Geometry: see drawing. Coordinates: mm, zero at the bounding-box minimum. A direction names the side the tool comes from. Give positions to 0.01 mm unless a question says otherwise; leave off trailing zeros. Write each loop counter-clockwise with the first axis right and the second up, starting at its lowest first coordinate (ties: lowest second). Pieces come first, ordered by that corner, then holes. Notation, with made-up numbers: (29, 16) -> (82, 16) arc R12 ccw to (82, 38) -> close; hole circle Ø10 at (-8, 52.25). An arc over 180 degrees is marked (long way). Use one line per item in the form item = value. Start each with the question number.
(1) Cut plane D-D, the plane z = 21.25. Output: boundary loops of the cut face in (x, y).
(2) Draft query along Z for the marked faces 4, 5 and 6. Return one class per face: pulls with the +Z half, pulls with the -Z half, needs draft (parallel to the pull), parting line crosses it, or undercut.
(3) Cut plane A-A, the plane z = 10.75. Output: boundary loops of the cut face in (x, y) (1 decimal).
(4) Cut plane C-C, the plane x = 18.75. Output: boundary loops of the cut face in (y, z) (1 decimal), and give its area (3 significant figures).
(5) Material intervals for line 1 along Y through (x, z) = (15, 23); line 2 along X through (y, z) = (4, 4) (1 decimal); line 3 along X through (y, z) = (6.25, 24.5), sorted ascending. Write a range as from..to.
(6) Cut plane B-B, the plane y = 8.75. Output: boundary loops of the cut face in (x, z) (1 decimal).
(7) Set-up query: the marked faces 1, 2 and 3. Return all of +Z, -Z, +X, -X, +Y, -Y with unobstructed straight access to the full face (end or side cutting, diameter ignored); none if empty.
(8) First-contact query: P1, Ø10, axis at x = 10.5, z = 24, coming from the +Y side; P2, Ø3, axis at x = 23, y = 2.5, coming from the +Z side; P3, Ø1.5, axis at x = 26.5, y = 7.5, coming from the -Z side (1 decimal). Flat tips, straight axial feed; report the tip coordinate or a pass-through.
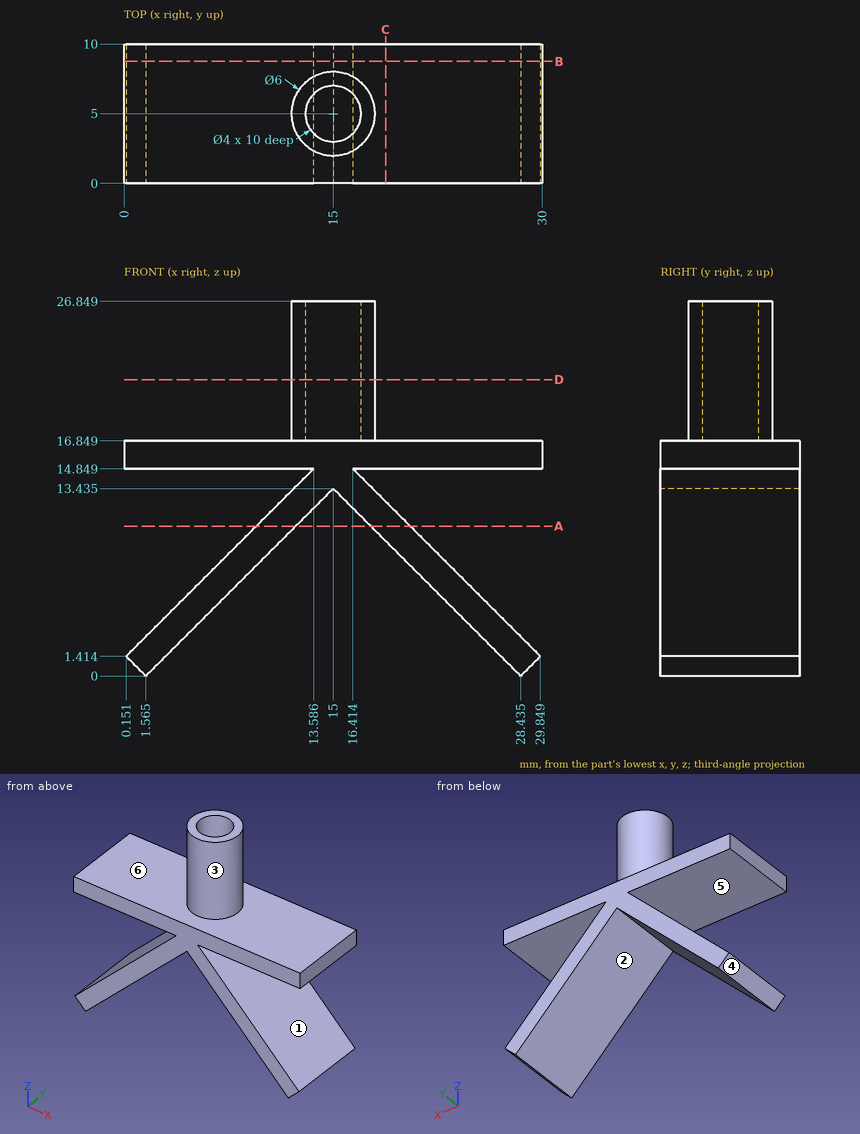
Geometry says:
q1.outline = circle Ø6 at (15, 5); hole circle Ø4 at (15, 5)
q2.face_4 = pulls with the -Z half
q2.face_5 = undercut
q2.face_6 = pulls with the +Z half
q3.outline = (9.5, 0) -> (12.3, 0) -> (12.3, 10) -> (9.5, 10) -> close; (17.7, 0) -> (20.5, 0) -> (20.5, 10) -> (17.7, 10) -> close
q4.outline = (0, 9.7) -> (10, 9.7) -> (10, 12.5) -> (0, 12.5) -> close; (0, 14.8) -> (10, 14.8) -> (10, 16.8) -> (0, 16.8) -> close
q4.area = 48.3 mm^2
q5.line_1 = 2..3, 7..8
q5.line_2 = 2.7..5.6, 24.4..27.3
q5.line_3 = 12.27..13.44, 16.56..17.73
q6.outline = (0, 14.8) -> (13.6, 14.8) -> (0.2, 1.4) -> (1.6, 0) -> (15, 13.4) -> (28.4, 0) -> (29.8, 1.4) -> (16.4, 14.8) -> (30, 14.8) -> (30, 16.8) -> (0, 16.8) -> close
q7.face_1 = +X, +Y, -Y
q7.face_2 = -Z, +Y, -Y
q7.face_3 = +Z
q8.P1 = 8
q8.P2 = 16.85
q8.P3 = 1.2
